```python
from build123d import *

# Parameters (mm, degrees)
CUT_EXTRUDE1_DEPTH      = 545.248334862
CUT_EXTRUDE1_DEPTH_BACK = 545.248334862
SKETCH2_R               = 8


with BuildPart() as part:
    # Sketch1 → Revolve1 (revolve)
    with BuildSketch(Plane.XY, mode=Mode.PRIVATE) as revolve1_sk:
        Polygon((-320, 586.81862199), (-320, 769.31862199), (-365, 769.31862199), (-365, 759.31862199), (-325, 759.31862199), (-325, 596.81862199), (-365, 596.81862199), (-365, 586.81862199), align=None)
    revolve(revolve1_sk.sketch.rotate(Axis((0, -8382.840526503, 0), (0, 1, 0)), 180), axis=Axis((0, -8382.840526503, 0), (0, 1, 0)))

    # Sketch2 → Cut-Extrude1 (cut, two sides: drawn at the far end of the back side and taken through both)
    with BuildSketch(Plane(origin=(0, 596.81862199, 0), x_dir=(1, 0, 0), z_dir=(0, 1, 0)).offset(-CUT_EXTRUDE1_DEPTH_BACK)):
        with Locations(Location((0, 345, 0), (0, 0, 180))):
            Circle(SKETCH2_R)
        with BuildLine():
            ThreePointArc((139.347363526, 315.514392242), (134.951947446, 325.802821793), (124.568900626, 321.635832007))
            ThreePointArc((124.568900626, 321.635832007), (128.964316707, 311.347402456), (139.347363526, 315.514392242))
        make_face()
        with Locations(Location((243.951839509, 243.951839509, 0), (0, 0, 180))):
            Circle(SKETCH2_R)
        with Locations(Location((318.738438716, 132.025784166, 0), (0, 0, 180))):
            Circle(SKETCH2_R)
        with Locations(Location((345, 0, 0), (0, 0, 180))):
            Circle(SKETCH2_R)
        with Locations(Location((318.738438716, -132.025784166, 0), (0, 0, 180))):
            Circle(SKETCH2_R)
        with Locations(Location((243.951839509, -243.951839509, 0), (0, 0, 180))):
            Circle(SKETCH2_R)
        with Locations(Location((132.025784166, -318.738438716, 0), (0, 0, 180))):
            Circle(SKETCH2_R)
        with Locations(Location((0, -345, 0), (0, 0, 180))):
            Circle(SKETCH2_R)
        with Locations(Location((-132.025784166, -318.738438716, 0), (0, 0, 180))):
            Circle(SKETCH2_R)
        with Locations(Location((-243.951839509, -243.951839509, 0), (0, 0, 180))):
            Circle(SKETCH2_R)
        with Locations(Location((-318.738438716, -132.025784166, 0), (0, 0, 180))):
            Circle(SKETCH2_R)
        with Locations(Location((-345, 0, 0), (0, 0, 180))):
            Circle(SKETCH2_R)
        with Locations(Location((-318.738438716, 132.025784166, 0), (0, 0, 180))):
            Circle(SKETCH2_R)
        with Locations(Location((-243.951839509, 243.951839509, 0), (0, 0, 180))):
            Circle(SKETCH2_R)
        with Locations(Location((-132.025784166, 318.738438716, 0), (0, 0, 180))):
            Circle(SKETCH2_R)
    extrude(amount=CUT_EXTRUDE1_DEPTH + CUT_EXTRUDE1_DEPTH_BACK, mode=Mode.SUBTRACT)


solid = part.part
```
The model under review builds one solid part; all positions refer to its coordinate system, in mm. A direction names the side the tool comes from. Round coordinates to 2 decimals unless told otherwise and drop trailing zeros. Loops run counter-clockwise (first coordinate to the right, second up) from the corner with the lowest first, then second, coordinate; pieces in that order, holes last. Notation, with made-up numbers: (40, 45) -> (48, 45) arc R13 ccw to (48, 70) -> close; hole circle Ø3 at (58, 53). An arc over 180 degrees is marked (long way). Answer as a JSON object with one key per item and string values. Group by question number.
1) We need section A-A on z = 105. Write out the cut boundary in (x, y).
2) We need section B-B on x = -188. Write out the cut boundary in (y, z).
3) Mouldability with a two-part tool opening along Y and no side actions: class faces 1 (the face through (-235.96, 591.75, -243.6)), 2 (the face through (218, 596.819, -245)) as released by +Y, released by -Y, zero draft, split by the parting line, or undercut.
4) For pin 1 Ø18.5 at (x, z) = (318.74, -132.03) entering from -Y; pin 2 Ø13 at (x, z) = (-345, 0) entering from +Y; pin 3 Ø1.5 at (y, z) = (661.5, 90) entering from +X; pin 4 Ø1.5 at (x, y) = (245.5, 635.5) entering from -Z, all flat-tipped, find the tip position at first contact; note any pin that passes through.
5) We need section C-C on y = 606. Write out the cut boundary in (x, z), then the cut area to 3 significant figures.
6) For line 1 (Z direction, x = 0, y = 591); line 2 (Z direction, x = 7.5, y = 751.5); line 3 (Z direction, x = 97.5, y = 635), list the stretches that pass through material, from the lowest coordinate up. Write a range as [from, to].
7) For faces 3 (the face through (310, 676.9, -97.6)), 4 (the face through (319.78, 764.249, -124.094)), list the 3-axis set-ups (+Z, -Z, +X, -X, +Y, -Y) from which the entire face can be reached by the end or side of a thin tool; tool diameter is ignored.
Result set:
{
 "1": {"outline": "(-349.57, 586.82) -> (-302.28, 586.82) -> (-302.28, 769.32) -> (-349.57, 769.32) -> (-349.57, 759.32) -> (-307.57, 759.32) -> (-307.57, 596.82) -> (-349.57, 596.82) -> close; (302.28, 586.82) -> (349.57, 586.82) -> (349.57, 596.82) -> (307.57, 596.82) -> (307.57, 759.32) -> (349.57, 759.32) -> (349.57, 769.32) -> (302.28, 769.32) -> close"},
 "2": {"outline": "(586.82, -312.86) -> (596.82, -312.86) -> (596.82, -265.11) -> (759.32, -265.11) -> (759.32, -312.86) -> (769.32, -312.86) -> (769.32, -258.95) -> (586.82, -258.95) -> close; (586.82, 258.95) -> (769.32, 258.95) -> (769.32, 312.86) -> (759.32, 312.86) -> (759.32, 265.11) -> (596.82, 265.11) -> (596.82, 312.86) -> (586.82, 312.86) -> close"},
 "3": {"face 1": "zero draft", "face 2": "undercut"},
 "4": {"pin 1": "y = 586.82", "pin 2": "through", "pin 3": "x = 312.51", "pin 4": "z = -213.83"},
 "5": {"outline": "circle Ø650 at (0, 0); hole circle Ø640 at (0, 0)", "area": "10,100 mm²"},
 "6": {"line 1": "[-365, -353], [-337, -320], [320, 337], [353, 365]", "line 2": "[-324.91, -319.91], [319.91, 324.91]", "line 3": "[-310.03, -304.78], [304.78, 310.03]"},
 "7": {"face 3": "none", "face 4": "+Y, -Y"}
}
